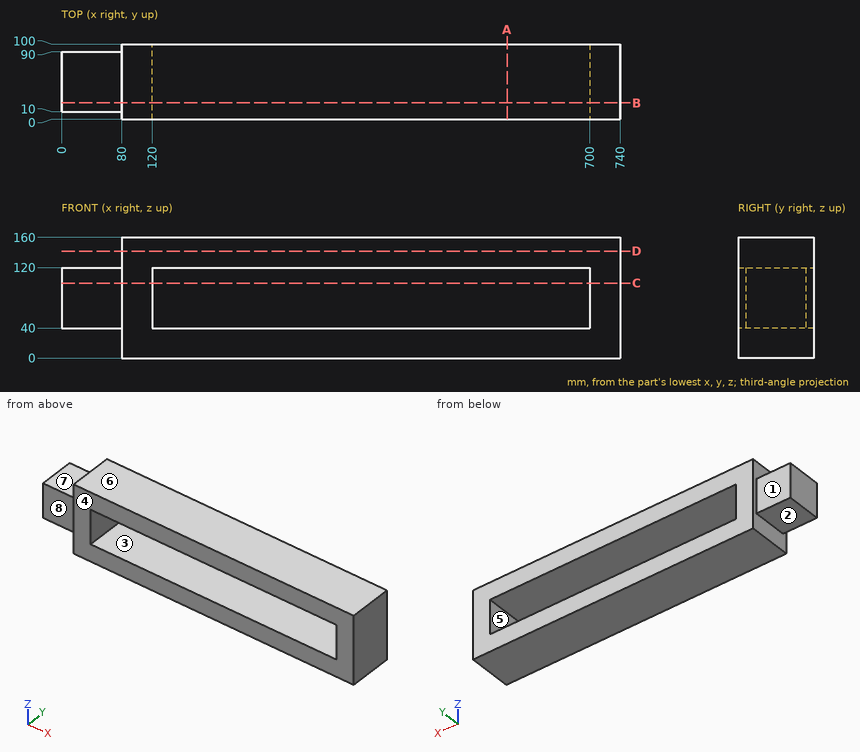
Verification items for this drawing (mm, ordinates from the low corner). A direction names the side the tool comes from. Coordinates: 2 decimals unless noted, no trailing zeros. Order: outer loops, then holes, each group sorted by start corner. A loop starts at its lowest first (then second) coordinate and runs counter-clockwise, first axis right, second up. Notation, with made-up numbers: (50, 57) -> (70, 57) arc R20 ccw to (70, 89) -> close; hole circle Ø6 at (76.25, -11). An arc over 180 degrees is marked (long way). Put each result on its own line as item: value. Start each with the question number.
1. Cross-section at D-D, the plane z = 142. Record the boundary of the cut face in (x, y), then the cut area to 3 significant figures.
2. Access from +Z, -Z, +X, -X, +Y, -Y to the whole of each face (thin tool, end or side, straight path). Record for the marked faces 4, 5, 6, 7 and 8.
3. Go/stop test with flat-tipped pins: pin 1 Ø24 at (x, y) = (26.5, 59) entering from +Z; pin 2 Ø3 at (y, z) = (67, 144) entering from -X. Record where each tip stops, or that it passes through.
4. Material ranges on L1, parallel to Z at x = 536, y = 52; L2, parallel to X at y = 60, z = 89; L3, parallel to X at y = 50.5, z = 136, recorded low to high. Write a range as [from, to].
5. Cross-section at A-A, the plane x = 590.5. Record the boundary of the cut face in (y, z).
6. Cross-section at C-C, the plane z = 99.5. Record the boundary of the cut face in (x, y), then the cut area to 3 significant figures.
7. Cross-section at B-B, the plane y = 22. Record the boundary of the cut face in (x, z).
8. Mould release check, pull along Z, two halves, no side actions. Record for the marked faces 1, 2 and 3: released by +Z, released by -Z, zero draft, split by the parting line, or undercut.
Computed:
1. outline: (80, 0) -> (740, 0) -> (740, 100) -> (80, 100) -> close
1. area: 66,000 mm2
2. face 4: +Z, -Z, +X, -X, -Y
2. face 5: +Y, -Y
2. face 6: +Z, +X, -X, +Y, -Y
2. face 7: +Z, -X, +Y, -Y
2. face 8: +Z, -Z, -X, -Y
3. pin 1: z = 120
3. pin 2: x = 80
4. L1: [0, 40], [120, 160]
4. L2: [0, 120], [700, 740]
4. L3: [80, 740]
5. outline: (0, 0) -> (100, 0) -> (100, 40) -> (0, 40) -> close; (0, 120) -> (100, 120) -> (100, 160) -> (0, 160) -> close
6. outline: (0, 10) -> (80, 10) -> (80, 0) -> (120, 0) -> (120, 100) -> (80, 100) -> (80, 90) -> (0, 90) -> close; (700, 0) -> (740, 0) -> (740, 100) -> (700, 100) -> close
6. area: 14,400 mm2
7. outline: (0, 40) -> (80, 40) -> (80, 0) -> (740, 0) -> (740, 160) -> (80, 160) -> (80, 120) -> (0, 120) -> close; hole (120, 40) -> (700, 40) -> (700, 120) -> (120, 120) -> close
8. face 1: zero draft
8. face 2: released by -Z
8. face 3: undercut
